from build123d import *

# Parameters (mm, degrees)
F0_R     = 1.5
F1_DEPTH = 7
F2_R     = 2
F3_DEPTH = 3
F4_W     = 2.5
F4_H     = 2.5
F5_DEPTH = 2


with BuildPart() as f1:
    # F0 (on Front) → F1 (new body)
    with BuildSketch(Plane.XZ):
        Circle(F0_R)
    extrude(amount=F1_DEPTH)

    # F2 (on face) → F3 (join)
    with BuildSketch(Plane.XZ.offset(7)):
        Circle(F2_R)
    extrude(amount=F3_DEPTH)

    # F4 (on face) → F5 (join)
    with BuildSketch(Plane.XZ.offset(10)):
        Rectangle(F4_W, F4_H)
    extrude(amount=F5_DEPTH)


solid = f1.part
Check sheet for the modelled part. Datum: model origin and axes. Units: mm. A direction names the side the tool comes from. Give positions to 0.01 mm unless a question says otherwise; leave off trailing zeros. Loops run counter-clockwise (first coordinate to the right, second up) from the corner with the lowest first, then second, coordinate; pieces in that order, holes last. Notation, with made-up numbers: M 72.25,37.25 L 107.25,37.25 A5 ccw 107.25,43.25 Z; hole C -14,57 d11. An arc over 180 degrees is marked long. Return JSON: item names as keys, results as strings. Group by question number.
1. Thickness scan on L1, parallel to Y at x = -1.6, z = 0.3; L2, parallel to Y at x = -1.1, z = 1.2; L3, parallel to X at y = -6, z = 0.1. Record the ranges inside material, lowest first.
2. Cross-section at D-D on y = -9.5. Record the boundary of the cut face in (x, z), plus the area to 3 significant figures.
3. Go/stop test with flat-tipped pins: pin 1 (2 mm diameter, centred on y = -11.5, z = -0.5, fed in from +X); pin 2 (0.6 mm diameter, centred on x = -0.5, y = -11, fed in from +Z); pin 3 (0.6 mm diameter, centred on x = 0.5, y = -11, fed in from -Z). Record where each tip stops, or that it passes through.
4. Tool access check on faces 1 (the flat face through (-1.25, -11, 0)), 2 (the flat face through (0, -11, -1.25)), 3 (the flat face through (0, -11, 1.25)), 4 (the cylindrical face through (-1.5, -3.45, 0.07)), 5 (the flat face through (1.25, -11, 0)). Record the directions out of +Z, -Z, +X, -X, +Y, -Y that give a thin tool (end or side, any length) a straight path to the whole face; none if there is none.
5. Cross-section at B-B on x = 0. Record the boundary of the cut face in (y, z).
6. Cross-section at C-C on y = -6.25. Record the boundary of the cut face in (x, z), plus the area to 3 significant figures.
7. Cross-section at A-A on z = 0. Record the boundary of the cut face in (x, y), plus the area to 3 significant figures.
Return value:
{
 "1": {"L1": "-10 to -7", "L2": "-12 to -7", "L3": "-1.5 to 1.5"},
 "2": {"outline": "C 0,0 d4", "area": "12.6 mm^2"},
 "3": {"pin 1": "x = 1.25", "pin 2": "z = 1.25", "pin 3": "z = -1.25"},
 "4": {"face 1": "+Z, -Z, -X, -Y", "face 2": "-Z, +X, -X, -Y", "face 3": "+Z, +X, -X, -Y", "face 4": "+Y", "face 5": "+Z, -Z, +X, -Y"},
 "5": {"outline": "M -12,-1.25 L -10,-1.25 L -10,-2 L -7,-2 L -7,-1.5 L 0,-1.5 L 0,1.5 L -7,1.5 L -7,2 L -10,2 L -10,1.25 L -12,1.25 Z"},
 "6": {"outline": "C 0,0 d3", "area": "7.07 mm^2"},
 "7": {"outline": "M -2,-10 L -1.25,-10 L -1.25,-12 L 1.25,-12 L 1.25,-10 L 2,-10 L 2,-7 L 1.5,-7 L 1.5,0 L -1.5,0 L -1.5,-7 L -2,-7 Z", "area": "38.0 mm^2"}
}
